Design review of the part shown in the three views and the two pictorial views. Dimensions are in mm from the part's minimum x, y and z. A direction names the side the tool comes from. Round coordinates to 2 decimals unless told otherwise and drop trailing zeros. Loops run counter-clockwise (first coordinate to the right, second up) from the corner with the lowest first, then second, coordinate; pieces in that order, holes last. Notation, with made-up numbers: (27.25, 21) -> (77.25, 21) arc R13 ccw to (77.25, 27) -> close; hole circle Ø10 at (-1, 81). An arc over 180 degrees is marked (long way). One line per question, with ' | ' between items. Start each with the question number.
1. Consider section D-D (y = 22.5). Write out the cut boundary in (x, z).
2. Consider section C-C (z = 145.5). Write out the cut boundary in (x, y).
3. Consider section A-A (y = 70). Write out the cut boundary in (x, z), and give its area (4 significant figures).
4. For pin 1 Ø2 at (x, z) = (79.5, 157) entering from +Y; pin 2 Ø12 at (y, z) = (39, 141) entering from -X; pin 3 Ø12 at (y, z) = (81.5, 214.5) entering from +X, all flat-tipped, find the tip position at first contact; note any pin that passes through.
5. For the marked faces 1 and 2, list the 3-axis set-ups (+Z, -Z, +X, -X, +Y, -Y) from which the entire face can be reached by the end or side of a thin tool; tool diameter is ignored.
6. Wall thickness on line 1 along Y through (x, z) = (70, 241); line 2 along X through (y, z) = (72, 50.5); line 3 along Z through (x, y) = (42.5, 55.5): over which ranges is each line inside the solid? List them lowest first.
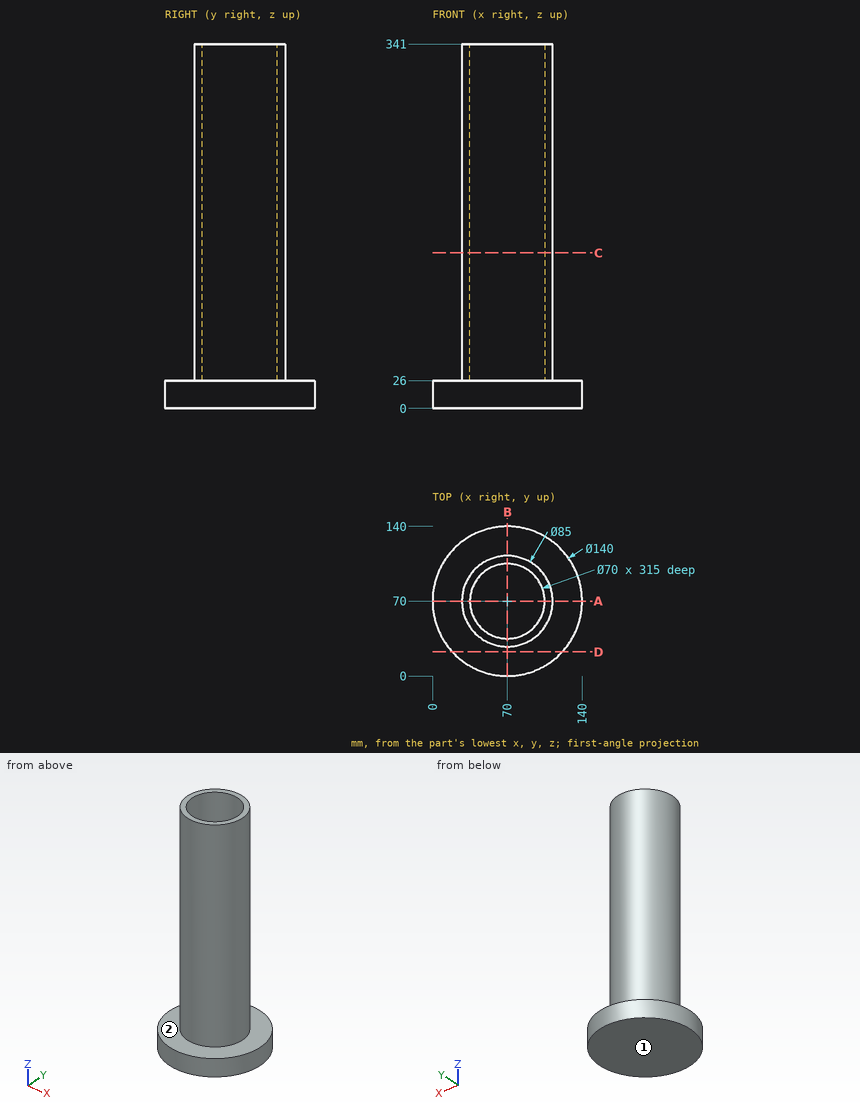
Answer block:
1) outline: (18.58, 0) -> (121.42, 0) -> (121.42, 26) -> (18.58, 26) -> close
2) outline: circle Ø85 at (70, 70); hole circle Ø70 at (70, 70)
3) outline: (0, 0) -> (140, 0) -> (140, 26) -> (112.5, 26) -> (112.5, 341) -> (105, 341) -> (105, 26) -> (35, 26) -> (35, 341) -> (27.5, 341) -> (27.5, 26) -> (0, 26) -> close | area: 8,365 mm2
4) pin 1: stops at y = 111.64 | pin 2: stops at x = 35.63 | pin 3: stops at x = 112.14
5) face 1: -Z, +X, -X, +Y, -Y | face 2: +Z
6) line 1: y = 27.5 to 35, 105 to 112.5 | line 2: x = 27.55 to 35.06, 104.94 to 112.45 | line 3: z = 0 to 26
